Could you check a few things on this model? Use its own coordinates, in mm. A direction names the side the tool comes from. Round coordinates to 2 decimals unless told otherwise and drop trailing zeros. Write each loop counter-clockwise with the first axis right and the second up, starting at its lowest first coordinate (ties: lowest second). Pieces come first, ordered by that corner, then holes. Notation, with made-up numbers: (1.25, 75.5) - (56.25, 75.5) arc R27 cw to (56.25, 98.5) - close; hole circle Ø7 at (50, 72.25). An arc over 180 degrees is marked (long way). Put each result on its own line as item: value.
from build123d import *

# Parameters (mm, degrees)
SALIENTE_EXTRUIR1_DEPTH = 12.5
CROQUIS3_R              = 7.5
SALIENTE_EXTRUIR2_DEPTH = 19.5
CROQUIS4_W              = 20
CROQUIS4_H              = 25
CORTAR_EXTRUIR1_DEPTH   = 12
CROQUIS5_W              = 20
CROQUIS5_H              = 25
CORTAR_EXTRUIR2_DEPTH   = 12
REDONDEO1_R             = 10
REDONDEO2_R             = 5
CROQUIS7_R              = 6
SALIENTE_EXTRUIR4_DEPTH = 7
SALIENTE_EXTRUIR5_START = 7
CROQUIS8_R              = 6
SALIENTE_EXTRUIR5_DEPTH = 7


with BuildPart() as part:
    # Croquis1 → Saliente-Extruir1 (new, symmetric)
    with BuildSketch(Plane.XY):
        with BuildLine():
            Line((4.147680169, -1.57927741), (-36.48467702, -1.57927741))
            ThreePointArc((-36.48467702, -1.57927741), (-40.58891874, -2.30296596), (-44.198128336, -4.386744092))
            Line((-44.198128336, -4.386744092), (-51.88666001, -10.838188184))
            ThreePointArc((-51.88666001, -10.838188184), (-55.048902138, -14.95930236), (-56.173208693, -20.030721501))
            Line((-56.173208693, -20.030721501), (-56.173208693, -23.839337705))
            ThreePointArc((-56.173208693, -23.839337705), (-55.048902138, -28.910756846), (-51.88666001, -33.031871023))
            Line((-51.88666001, -33.031871023), (-44.198128336, -39.483315114))
            ThreePointArc((-44.198128336, -39.483315114), (-40.58891874, -41.567093246), (-36.48467702, -42.290781797))
            Line((-36.48467702, -42.290781797), (4.147680169, -42.290781797))
            Line((4.147680169, -42.290781797), (4.147680169, -1.57927741))
        make_face()
    extrude(amount=SALIENTE_EXTRUIR1_DEPTH, both=True)

    # Croquis3 → Saliente-Extruir2 (add, symmetric)
    with BuildSketch(Plane.XY):
        with Locations((-46.173208693, -22.290781797)):
            Circle(CROQUIS3_R)
    extrude(amount=SALIENTE_EXTRUIR2_DEPTH, both=True)

    # Croquis4 → Cortar-Extruir1 (cut)
    with BuildSketch(Plane(origin=(0, -1.57927741, 0), x_dir=(1, 0, 0), z_dir=(0, 1, 0))):
        with Locations((-5.852319831, 0)):
            Rectangle(CROQUIS4_W, CROQUIS4_H)
    extrude(amount=-CORTAR_EXTRUIR1_DEPTH, mode=Mode.SUBTRACT)

    # Croquis5 → Cortar-Extruir2 (cut)
    with BuildSketch(Plane.XZ.offset(42.290781797)):
        with Locations((-5.852319831, 0)):
            Rectangle(CROQUIS5_W, CROQUIS5_H)
    extrude(amount=-CORTAR_EXTRUIR2_DEPTH, mode=Mode.SUBTRACT)

    # Redondeo1
    redondeo1_edges = [part.edges().sort_by_distance(p)[0] for p in [
        (-15.852319831, -1.57927741, 0),
        (-15.852319831, -42.290781797, 0),
    ]]
    fillet(redondeo1_edges, radius=REDONDEO1_R)

    # Redondeo2
    redondeo2_edges = [part.edges().sort_by_distance(p)[0] for p in [
        (-15.852319831, -13.57927741, 0),
        (-15.852319831, -30.290781797, 0),
    ]]
    fillet(redondeo2_edges, radius=REDONDEO2_R)

    # Croquis7 → Saliente-Extruir4 (add)
    with BuildSketch(Plane(origin=(0, -13.57927741, 0), x_dir=(1, 0, 0), z_dir=(0, 1, 0))):
        with Locations(Location((-3.502319831, 0, 0), (0, 0, 180))):
            Circle(CROQUIS7_R)
    extrude(amount=SALIENTE_EXTRUIR4_DEPTH)

    # Croquis8 → Saliente-Extruir5 (add)
    with BuildSketch(Plane.XZ.offset(30.290781797).offset(SALIENTE_EXTRUIR5_START)):
        with Locations(Location((-3.502319831, 0, 0), (0, 0, 180))):
            Circle(CROQUIS8_R)
    extrude(amount=-SALIENTE_EXTRUIR5_DEPTH)


solid = part.part
(1) For faces 1 (the face through (-53.666, -21.961, 16.049)), 2 (the face through (-53.666, -21.961, -15.951)), 3 (the face through (-5, -13.579, -6)), which set-ups out of +Z, -Z, +X, -X, +Y, -Y let a thin tool reach every point of the face, with its end or its side?
Values found:
face 1: +Z
face 2: -Z
face 3: +Y
(2) Imagine slicing it at B-B, the plane x = -41.5. List the corners of the cut face in (y, z) for me.
Values found:
outline: (-41.19, -12.5) - (-28.16, -12.5) - (-28.16, -19.5) - (-16.42, -19.5) - (-16.42, -12.5) - (-2.68, -12.5) - (-2.68, 12.5) - (-16.42, 12.5) - (-16.42, 19.5) - (-28.16, 19.5) - (-28.16, 12.5) - (-41.19, 12.5) - close
(3) Please list where these lines run through material, in increasing order: probe 1 along Z at (x, y) = (-30, -8); probe 2 along Y at (x, z) = (-4.5, -4); probe 3 along Y at (x, z) = (-3, -9.5). Write a range as from..to.
Values found:
probe 1: z = -12.5..12.5
probe 2: y = -37.29..-6.58
probe 3: y = -30.29..-13.58
(4) Imagine slicing it at C-C, the plane x = -24. List the corners of the cut face in (y, z) for me, then the cut area to 3 significant figures.
Values found:
outline: (-42.12, -12.5) - (-1.75, -12.5) - (-1.75, 12.5) - (-42.12, 12.5) - close
area: 1,010 mm^2
(5) I'm going to push flat-ended pins straight in: pin 1 (4 mm diameter, centred on x = -3, z = -5.5, fed in from +Y); pin 2 (5 mm diameter, centred on x = -49.5, z = -10.5, fed in from +Y); pin 3 (6 mm diameter, centred on x = -18.5, y = -21, fed in from +Z); pin 4 (5 mm diameter, centred on y = -24.5, z = -6, fed in from -X). Where does each tip first touch, or does it pass through?
Values found:
pin 1: stops at y = -6.58
pin 2: stops at y = -6.74
pin 3: stops at z = 12.5
pin 4: stops at x = -56.17
(6) Imagine slicing it at A-A, the plane y = -17. List the corners of the cut face in (x, z) for me.
Values found:
outline: (-55.78, -12.5) - (-51.49, -12.5) - (-51.49, -19.5) - (-40.86, -19.5) - (-40.86, -12.5) - (4.15, -12.5) - (4.15, 12.5) - (-40.86, 12.5) - (-40.86, 19.5) - (-51.49, 19.5) - (-51.49, 12.5) - (-55.78, 12.5) - close
